Work out the finished part from the listing and answer in its coordinate system (mm). A direction names the side the tool comes from. Coordinates: 2 decimals unless noted, no trailing zeros. Order: outer loops, then holes, each group sorted by start corner. A loop starts at its lowest first (then second) coordinate and runs counter-clockwise, first axis right, second up.
```python
from build123d import *

# Parameters (mm, degrees)
F1_DEPTH = 15
F2_W     = 23
F2_H     = 11
F3_DEPTH = 4
F4_W     = 1
F4_H     = 11
F5_DEPTH = 4


with BuildPart() as f1:
    # F0 (on Front) → F1 (new body)
    with BuildSketch(Plane.XZ):
        Polygon((-6.555008, 5), (-11.455226, 0), (11.544774, 0), (6.644992, 5), align=None)
    extrude(amount=F1_DEPTH)

    # F2 (on face) → F3 (cut)
    with BuildSketch(Plane.XY.offset(5)):
        with Locations((0.044774, -7.5)):
            Rectangle(F2_W, F2_H)
    extrude(amount=-F3_DEPTH, mode=Mode.SUBTRACT)

    # F4 (on face) → F5 (join)
    with BuildSketch(Plane.XY.offset(1)):
        with Locations((0.044818, -7.5)):
            Rectangle(F4_W, F4_H)
    extrude(amount=F5_DEPTH)


solid = f1.part
```
1. The part is cut by section B-B (y = -6.5). Determine the outline of the cut face in (x, z).
2. Flat-ended cylindrical pins translate along their axes: pin 1 (3 mm diameter, centred on x = 7.5, y = -8, fed in from +Z); pin 2 (2 mm diameter, centred on y = -12.5, z = 2.5, fed in from +X); pin 3 (1.2 mm diameter, centred on y = -6.5, z = 4, fed in from +X). Find the tip coordinate at first contact, or state that the pin passes through.
3. For faces 5 (the flat face through (-10.6, -7.4, 0.87)), 6 (the flat face through (-0.455, -8, 3)), 7 (the flat face through (5, -7, 1)), determine the directions among +Z, -Z, +X, -X, +Y, -Y from which every point of the face is accessible in a straight line to the end or side of a thin tool.
4. The mould has two halves that part along Y. Classify faces 1 (the flat face through (-4, -13, 3)), 2 (the flat face through (0, -15, 3)), 3 (the flat face through (-4, -2, 3)), 4 (the flat face through (0, -7, 0)): released by +Y, released by -Y, zero draft, split by the parting line, or undercut.
5. The part is cut by section A-A (x = -5.5). Determine the outline of the cut face in (y, z).
6. Consider probe 1 along Y at (x, z) = (-6.75, 2); probe 2 along Z at (x, y) = (-7.5, -9.25); probe 3 along X at (y, z) = (-5, 3.8). Determine where each line is inside the solid, lowest interval first.
7. The part is cut by section D-D (z = 4.1). Determine the outline of the cut face in (x, y), plus the area to 3 significant figures.
8. The part is cut by section C-C (z = 3). Determine the outline of the cut face in (x, y).
Worked out:
1. outline: (-11.46, 0) - (11.54, 0) - (10.56, 1) - (0.54, 1) - (0.54, 5) - (-0.46, 5) - (-0.46, 1) - (-10.48, 1) - close
2. pin 1: stops at z = 1
2. pin 2: stops at x = 9.94
2. pin 3: stops at x = 0.54
3. face 5: +Z, -X, +Y, -Y
3. face 6: +Z, -X
3. face 7: +Z, +X
4. face 1: undercut
4. face 2: released by -Y
4. face 3: undercut
4. face 4: zero draft
5. outline: (-15, 0) - (0, 0) - (0, 5) - (-2, 5) - (-2, 1) - (-13, 1) - (-13, 5) - (-15, 5) - close
6. probe 1: y = -15 to -13, -2 to 0
6. probe 2: z = 0 to 1
6. probe 3: x = -0.46 to 0.54
7. outline: (-7.44, -15) - (7.53, -15) - (7.53, -13) - (0.54, -13) - (0.54, -2) - (7.53, -2) - (7.53, 0) - (-7.44, 0) - (-7.44, -2) - (-0.46, -2) - (-0.46, -13) - (-7.44, -13) - close
7. area: 70.9 mm2
8. outline: (-8.52, -15) - (8.6, -15) - (8.6, -13) - (0.54, -13) - (0.54, -2) - (8.6, -2) - (8.6, 0) - (-8.52, 0) - (-8.52, -2) - (-0.46, -2) - (-0.46, -13) - (-8.52, -13) - close
